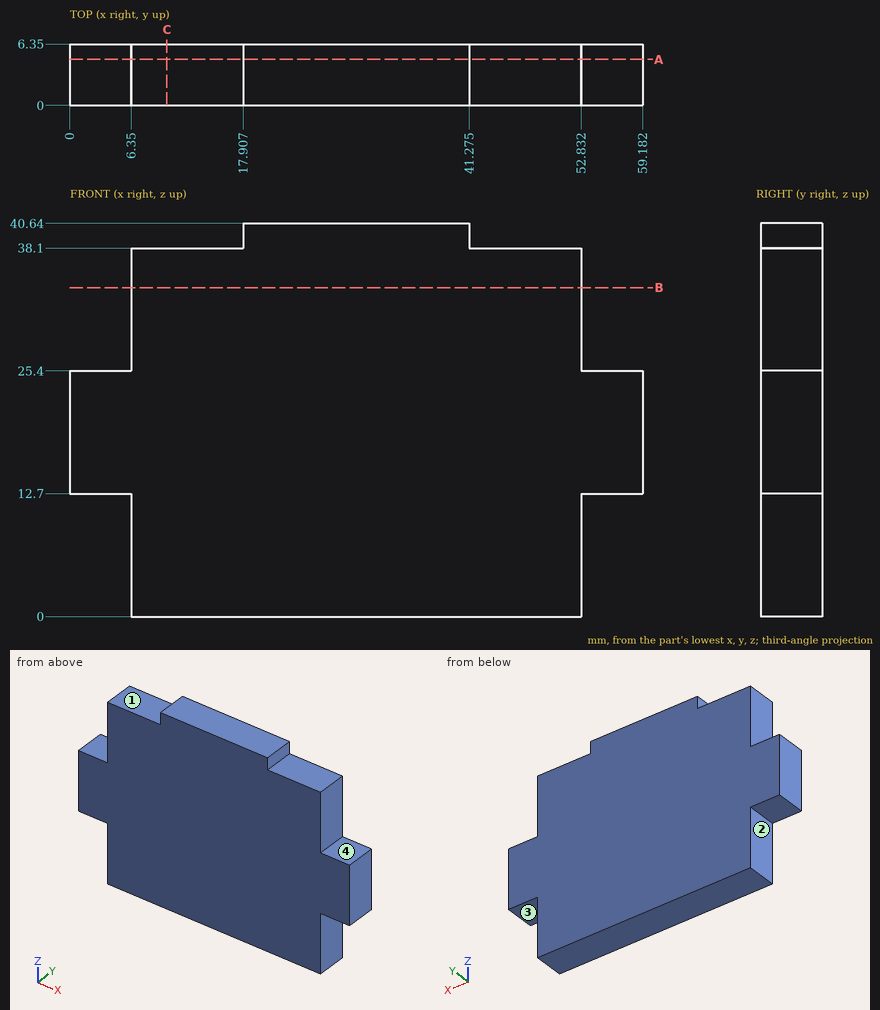
Geometry check sheet. Reference: drawing and pictorial views, mm from the part's lowest x, y, z. A direction names the side the tool comes from. Round coordinates to 2 decimals unless told otherwise and drop trailing zeros. Order: outer loops, then holes, each group sorted by start corner. A loop starts at its lowest first (then second) coordinate and runs counter-clockwise, first axis right, second up. Notation, with made-up numbers: (17, 21.5) - (59, 21.5) arc R10 ccw to (59, 36.5) - close; hole circle Ø6 at (-16.5, -12). An arc over 180 degrees is marked (long way). One line per question, with ' | ' between items. Start each with the question number.
(1) Sectioned sample at C-C on x = 10. Record the cut outline in (y, z), and give its area (3 significant figures).
(2) Sectioned sample at A-A on y = 4.75. Record the cut outline in (x, z) (3 decimals).
(3) Access from +Z, -Z, +X, -X, +Y, -Y to the whole of each face (thin tool, end or side, straight path). Record for the marked faces 1, 2, 3 and 4.
(4) Sectioned sample at B-B on z = 34. Record the cut outline in (x, y).
(5) Thickness scan on L1, parallel to Z at x = 57.5, y = 3; L2, parallel to X at y = 3.5, z = 8.5; L3, parallel to Z at x = 11.5, y = 4.25. Record the ranges inside material, lowest first. Write a range as [from, to].
(6) Depth check by flat-ended pin: pin 1 Ø3 at (x, y) = (54.5, 3.5) entering from -Z; pin 2 Ø1 at (y, z) = (2.5, 8) entering from -X; pin 3 Ø1.3 at (y, z) = (3, 39) entering from -X. Enter the tip coordinate at first touch or a pass-through.
Conclusion:
1) outline: (0, 0) - (6.35, 0) - (6.35, 38.1) - (0, 38.1) - close | area: 242 mm2
2) outline: (0, 12.7) - (6.35, 12.7) - (6.35, 0) - (52.832, 0) - (52.832, 12.7) - (59.182, 12.7) - (59.182, 25.4) - (52.832, 25.4) - (52.832, 38.1) - (41.275, 38.1) - (41.275, 40.64) - (17.907, 40.64) - (17.907, 38.1) - (6.35, 38.1) - (6.35, 25.4) - (0, 25.4) - close
3) face 1: +Z, -X, +Y, -Y | face 2: -Z, -X, +Y, -Y | face 3: -Z, +X, +Y, -Y | face 4: +Z, +X, +Y, -Y
4) outline: (6.35, 0) - (52.83, 0) - (52.83, 6.35) - (6.35, 6.35) - close
5) L1: z = [12.7, 25.4] | L2: x = [6.35, 52.83] | L3: z = [0, 38.1]
6) pin 1: stops at z = 12.7 | pin 2: stops at x = 6.35 | pin 3: stops at x = 17.91
